Geometry: final body of the model. Coordinates: model frame, mm. A direction names the side the tool comes from. Round coordinates to 2 decimals unless told otherwise and drop trailing zeros. Write each loop counter-clockwise with the first axis right and the second up, starting at its lowest first coordinate (ties: lowest second). Pieces come first, ordered by that corner, then holes. Notation, with made-up numbers: M 37,-18.75 L 76,-18.75 A16 cw 76,11.25 Z; hole C 6.25,-5 d11. An arc over 180 degrees is marked long. Use one line per item in the form item = value. Start each with the question number.
Item 1: Pin query (flat end, axial travel): pin 1 Ø4 at (x, z) = (3, 63.5) entering from -Y; pin 2 Ø1 at (x, z) = (3, 110) entering from -Y; pin 3 Ø2 at (y, z) = (-3.5, 73.5) entering from +X. Return the tip coordinate at first contact, or that it passes through.
Item 2: Section query A-A (x = 0). Return loops of the section in (y, z).
Item 3: Reachability of faces 1 (the flat face through (0, 4.9, 145)), 2 (the flat face through (0, -4.9, 145)), 3 (the cylindrical face through (-6, 0, 79)) from +Z, -Z, +X, -X, +Y, -Y: full face, straight path, thin tool, end or side. Return the list, or none.
Item 4: Section query D-D (z = 135). Return loops of the section in (x, y).
Item 5: Section query B-B (z = 59). Return loops of the section in (x, y), and give its area (3 significant figures).
Item 6: Section query C-C (y = 2.75). Return loops of the section in (x, z), and give its area (3 significant figures).
Item 7: Ray query, probe 1 along Y at (x, z) = (-3.5, 68.5); probe 2 along X at (y, z) = (2.5, 98.5); probe 3 along X at (y, z) = (5, 70). Return the intervals inside material, ascending.
Autodesk Inventor part; units mm, degrees
ref_plane "YZ Plane" through (0, 0, 0) normal (1, 0, 0) x (0, 1, 0)
ref_plane "XZ Plane" through (0, 0, 0) normal (0, 1, 0) x (-1, 0, 0)
ref_plane "XY Plane" through (0, 0, 0) normal (0, 0, 1) x (1, 0, 0)
sketch "Sketch1" plane through (0, 0, 0) normal (0, 0, 1) x (1, 0, 0)
  circle A0 centre (0, 0) radius 6
  dimension "d0" = 12
extrude "Extrusion1" add sketch "Sketch1" along normal blind 160
sketch "Sketch2" plane through (0, 0, 160) normal (0, 0, 1) x (1, 0, 0)
  arc A0 (-3.4627, 4.9) -> (-3.4627, -4.9) centre (0, 0) ccw
  line L0 (-3.4627, 4.9) -> (3.4627, 4.9)
  arc A1 (3.4627, -4.9) -> (3.4627, 4.9) centre (0, 0) ccw
  line L1 (3.4627, -4.9) -> (-3.4627, -4.9)
  line L2 (-4.1729, 7.0025) -> (4.0866, 7.0025)
  line L3 (4.0866, 7.0025) -> (4.0866, 4.9)
  line L4 (4.0866, 4.9) -> (-4.1729, 4.9)
  line L5 (-4.1729, 4.9) -> (-4.1729, 7.0025)
  line L6 (-3.9468, -4.9) -> (4.2356, -4.9)
  line L7 (4.2356, -4.9) -> (4.2356, -6.7965)
  line L8 (4.2356, -6.7965) -> (-3.9468, -6.7965)
  line L9 (-3.9468, -6.7965) -> (-3.9468, -4.9)
  point P0 (-3.4627, 4.9)
  point P1 (3.4627, -4.9)
  point P2 (-3.4627, -4.9)
extrude "Extrusion2" cut sketch "Sketch2" against normal blind 30 contours L4 L5 L2 L3 L0 | L1 L6 L7 L8 L9
properties part number "oś napędowa 12mm"
Working result:
q1.pin_1 = -5.92
q1.pin_2 = -5.45
q1.pin_3 = 5.45
q2.outline = M -6,0 L 6,0 L 6,130 L 4.9,130 L 4.9,160 L -4.9,160 L -4.9,130 L -6,130 Z
q3.face_1 = +Z, +X, -X, +Y
q3.face_2 = +Z, +X, -X, -Y
q3.face_3 = +Z, -Z
q4.outline = M -3.46,-4.9 L 3.46,-4.9 A6 ccw 3.46,4.9 L -3.46,4.9 A6 ccw Z
q5.outline = C 0,0 d12
q5.area = 113 mm²
q6.outline = M -5.33,0 L 5.33,0 L 5.33,160 L -5.33,160 Z
q6.area = 1,710 mm²
q7.probe_1 = -4.87 to 4.87
q7.probe_2 = -5.45 to 5.45
q7.probe_3 = -3.32 to 3.32
